```python
from build123d import *

# Parameters (mm, degrees)
F0_R     = 4.7625
F1_DEPTH = 6.35
F1_TAPER = 5
F2_R     = 3.175
F3_DEPTH = 19.05
F4_R     = 1.651
F5_DEPTH = 12.7
F6_SIZE  = 1.27
F7_R     = 0.762
F9_DEPTH = 4.445
F10_R    = 1.2699


# Not quite as in the source:
# - a fillet or chamfer is up to 0.001 mm smaller than in the source, because OpenCascade refuses the exact size
# - after a boolean that leaves OpenCascade's solid faulty, fix() repairs it


with BuildPart() as f1:
    # F0 (on Front) → F1 (new body)
    with BuildSketch(Plane.XZ):
        Circle(F0_R)
    extrude(amount=-F1_DEPTH, taper=F1_TAPER)

    # F2 (on face) → F3 (join)
    with BuildSketch(Plane.XZ):
        Circle(F2_R)
    extrude(amount=F3_DEPTH)

    # F4 (on face) → F5 (cut)
    with BuildSketch(Plane(origin=(0, 6.35, 0), x_dir=(-1, 0, 0), z_dir=(0, 1, 0))):
        Circle(F4_R)
    extrude(amount=-F5_DEPTH, mode=Mode.SUBTRACT)

    # F6
    f6_edges = [f1.edges().sort_by_distance(p)[0] for p in [
        (-3.175, -19.05, 0),
    ]]
    chamfer(f6_edges, length=F6_SIZE)

    # F7
    f7_edges = [f1.edges().sort_by_distance(p)[0] for p in [
        (-4.206947, 6.35, 0),
    ]]
    fillet(f7_edges, radius=F7_R)

    # F8 (on face) → F9 (cut)
    with BuildSketch(Plane.XZ):
        with BuildLine():
            ThreePointArc((-2.9099355663, -1.27), (-3.175, 0), (-2.9099355663, 1.27))
            Line((-2.9099355663, 1.27), (-4.5900442536, 1.27))
            ThreePointArc((-4.5900442536, 1.27), (-4.7625, 0), (-4.5900442536, -1.27))
            Line((-4.5900442536, -1.27), (-2.9099355663, -1.27))
        make_face()
    extrude(amount=-F9_DEPTH, mode=Mode.SUBTRACT)

    add(f1.part.fix(), mode=Mode.REPLACE)

    # F10 (radius 1.27 in the source; OpenCascade refuses exactly that, so slightly less here)
    f10_edges = [f1.edges().sort_by_distance(p)[0] for p in [
        (-3.547549, 4.445, 1.27),
        (-3.547549, 4.445, -1.27),
    ]]
    fillet(f10_edges, radius=F10_R)


solid = f1.part
```
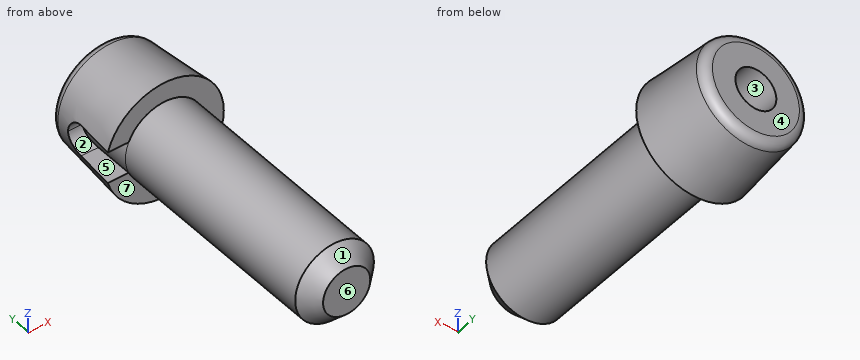
Verification items for the finished model (mm, model axes). Face numbers are marked on the shaded views. A direction names the side the tool comes from. Coordinates: 2 decimals unless noted, no trailing zeros. Loops run counter-clockwise (first coordinate to the right, second up) from the corner with the lowest first, then second, coordinate; pieces in that order, holes last. Notation, with made-up numbers: (19.5, 58) - (26.5, 58) arc R25 cw to (26.5, 95) - close; hole circle Ø9 at (12.5, 24.5). An arc over 180 degrees is marked (long way). Put each result on its own line as item: value.
Item 1: Gauge pin test, flat ends, axial feed: pin 1 Ø1 at (x, z) = (-2.5, -3.5) entering from -Y; pin 2 Ø2 at (x, z) = (0, 0) entering from +Y; pin 3 Ø5 at (y, z) = (-3.5, 0.5) entering from -X (3 decimals). Record the tip position at first contact, or that the pin passes through.
Conclusion:
pin 1: stops at y = 0
pin 2: stops at y = -6.35
pin 3: stops at x = -3.175
Item 2: Section check A-A (y = -4.5). Enter the section's corners in (x, z) (3 decimals).
Conclusion:
outline: circle Ø6.35 at (0, 0); hole circle Ø3.302 at (0, 0)
Item 3: Scan lines: line 1 along Z through (x, y) = (0, -0.5) (3 decimals); line 2 along Z through (x, y) = (-0.25, -5); line 3 along X through (y, z) = (2.75, 0.25) (3 decimals). Record each from-to range of solid material in increasing order.
Conclusion:
line 1: z = -3.175 to -1.651, 1.651 to 3.175
line 2: z = -3.17 to -1.63, 1.63 to 3.17
line 3: x = -3.165 to -1.632, 1.632 to 4.515
Item 4: Draft check along Z on the marked faces 1, 2, 3 and 4. Enter one of: pulls with the +Z half, pulls with the -Z half, needs draft (parallel to the pull), parting line crosses it, or undercut.
Conclusion:
face 1: parting line crosses it
face 2: undercut
face 3: undercut
face 4: needs draft
Item 5: Set-up check for the marked faces 5, 6 and 7: record each of +Z, -Z, +X, -X, +Y, -Y from which the full face is reachable in a straight line by a thin tool's end or side.
Conclusion:
face 5: -X, -Y
face 6: +Z, -Z, +X, -X, -Y
face 7: -Y
Item 6: Section check C-C (y = -11). Enter the section's corners in (x, z) (3 decimals), then the cut area to 3 significant figures.
Conclusion:
outline: circle Ø6.35 at (0, 0)
area: 31.7 mm2
